Part model, mm, in its own coordinate system. A direction names the side the tool comes from. Give positions to 0.01 mm unless a question says otherwise; leave off trailing zeros. Order: outer loops, then holes, each group sorted by start corner. A loop starts at its lowest first (then second) coordinate and runs counter-clockwise, first axis right, second up. Notation, with made-up numbers: M 69.25,10 L 94.25,10 A13 cw 94.25,17 Z; hole C 74,31.5 d8. An arc over 180 degrees is marked long. Answer as a JSON object with one key per item and string values.
from build123d import *

# Parameters (mm, degrees)
F1_DEPTH = 19.05


with BuildPart() as f1:
    # F0 (on Front) → F1 (new body)
    with BuildSketch(Plane.XZ):
        with BuildLine():
            Line((-159.199445, -158.121514), (107.500555, -158.121514))
            ThreePointArc((107.500555, -158.121514), (111.990683, -156.261642), (113.850555, -151.771514))
            Line((113.850555, -151.771514), (113.850555, 114.928486))
            ThreePointArc((113.850555, 114.928486), (111.990683, 119.418614), (107.500555, 121.278486))
            Line((107.500555, 121.278486), (-159.199445, 121.278486))
            ThreePointArc((-159.199445, 121.278486), (-163.689573, 119.418614), (-165.549445, 114.928486))
            Line((-165.549445, 114.928486), (-165.549445, -151.771514))
            ThreePointArc((-165.549445, -151.771514), (-163.689573, -156.261642), (-159.199445, -158.121514))
        make_face()
        with BuildLine():
            Line((-121.099445, -145.421514), (-146.499445, -145.421514))
            ThreePointArc((-146.499445, -145.421514), (-150.989573, -143.561642), (-152.849445, -139.071514))
            Line((-152.849445, -139.071514), (-152.849445, -113.671514))
            Line((-152.849445, -113.671514), (-152.849445, -81.921514))
            Line((-152.849445, -81.921514), (-152.849445, -50.171514))
            Line((-152.849445, -50.171514), (-152.849445, -18.421514))
            Line((-152.849445, -18.421514), (-152.849445, 13.328486))
            Line((-152.849445, 13.328486), (-152.849445, 45.078486))
            Line((-152.849445, 45.078486), (-152.849445, 76.828486))
            Line((-152.849445, 76.828486), (-152.849445, 102.228486))
            ThreePointArc((-152.849445, 102.228486), (-150.989573, 106.718614), (-146.499445, 108.578486))
            Line((-146.499445, 108.578486), (-121.099445, 108.578486))
            Line((-121.099445, 108.578486), (-89.349445, 108.578486))
            Line((-89.349445, 108.578486), (-57.599445, 108.578486))
            Line((-57.599445, 108.578486), (-25.849445, 108.578486))
            Line((-25.849445, 108.578486), (5.900555, 108.578486))
            Line((5.900555, 108.578486), (37.650555, 108.578486))
            Line((37.650555, 108.578486), (69.400555, 108.578486))
            Line((69.400555, 108.578486), (94.800555, 108.578486))
            ThreePointArc((94.800555, 108.578486), (99.290683, 106.718614), (101.150555, 102.228486))
            Line((101.150555, 102.228486), (101.150555, 76.828486))
            Line((101.150555, 76.828486), (101.150555, 45.078486))
            Line((101.150555, 45.078486), (101.150555, 13.328486))
            Line((101.150555, 13.328486), (101.150555, -18.421514))
            Line((101.150555, -18.421514), (101.150555, -50.171514))
            Line((101.150555, -50.171514), (101.150555, -81.921514))
            Line((101.150555, -81.921514), (101.150555, -113.671514))
            Line((101.150555, -113.671514), (101.150555, -139.071514))
            ThreePointArc((101.150555, -139.071514), (99.290683, -143.561642), (94.800555, -145.421514))
            Line((94.800555, -145.421514), (69.400555, -145.421514))
            Line((69.400555, -145.421514), (37.650555, -145.421514))
            Line((37.650555, -145.421514), (5.900555, -145.421514))
            Line((5.900555, -145.421514), (-25.849445, -145.421514))
            Line((-25.849445, -145.421514), (-57.599445, -145.421514))
            Line((-57.599445, -145.421514), (-89.349445, -145.421514))
            Line((-89.349445, -145.421514), (-121.099445, -145.421514))
        make_face(mode=Mode.SUBTRACT)
    extrude(amount=F1_DEPTH)


solid = f1.part
1. Which spindle directions (+Z, -Z, +X, -X, +Y, -Y) get a long thin tool onto all of the face, cutting with end or side? Do faces 4 (the cylindrical face through (99.24, -9.39, 106.77)), 5 (the flat face through (-24, -9, 121.278)). Say none if no direction does.
Worked answers:
{"face 4": "+Y, -Y", "face 5": "+Z, +X, -X, +Y, -Y"}
2. Cut at C-C on x = 38. Give the cut face in (y, z).
Worked answers:
{"outline": "M -19.05,-158.12 L 0,-158.12 L 0,-145.42 L -19.05,-145.42 Z; M -19.05,108.58 L 0,108.58 L 0,121.28 L -19.05,121.28 Z"}
3. Probe line 1 along Z through (x, y) = (63.5, -15.75); line 2 along X through (y, z) = (-10, -107). List the from-to ranges inside material, lowest first.
Worked answers:
{"line 1": "z = -158.12 to -145.42, 108.58 to 121.28", "line 2": "x = -165.55 to -152.85, 101.15 to 113.85"}
4. Cut at B-B on y = -14. Give the cut face in (x, z), plus the area to 3 significant figures.
Worked answers:
{"outline": "M -165.55,-151.77 A6.35 ccw -159.2,-158.12 L 107.5,-158.12 A6.35 ccw 113.85,-151.77 L 113.85,114.93 A6.35 ccw 107.5,121.28 L -159.2,121.28 A6.35 ccw -165.55,114.93 Z; hole M -152.85,-139.07 A6.35 ccw -146.5,-145.42 L 94.8,-145.42 A6.35 ccw 101.15,-139.07 L 101.15,102.23 A6.35 ccw 94.8,108.58 L -146.5,108.58 A6.35 ccw -152.85,102.23 Z", "area": "13,500 mm^2"}
5. Two-plate mould, pull along X, no slides. Class faces 1 (the flat face through (113.851, -9, -20)), 2 (the flat face through (-28, -9, 108.578)), 3 (the flat face through (-28, -9, -158.122)): +X half, -X half, draft (parallel to the pull), parting line (faces both ways), or undercut.
Worked answers:
{"face 1": "+X half", "face 2": "undercut", "face 3": "draft"}
6. Cut at A-A on z = 55. Give the cut face in (x, y).
Worked answers:
{"outline": "M -165.55,-19.05 L -152.85,-19.05 L -152.85,0 L -165.55,0 Z; M 101.15,-19.05 L 113.85,-19.05 L 113.85,0 L 101.15,0 Z"}
